Here's how the part is built. I have some questions about the finished solid (model axes, mm). A direction names the side the tool comes from. Give positions to 0.01 mm unless a question says otherwise; leave off trailing zeros. Write each loop counter-clockwise with the first axis right and the second up, starting at its lowest first coordinate (ties: lowest second). Pieces come first, ordered by that corner, then holes. Notation, with made-up numbers: M -39.75,44 L -14.75,44 A9 ccw -14.75,58 Z; hole C -9.75,5.5 d10. An arc over 180 degrees is marked long. Answer as CSV lines item,"result". Start each with the question number.
Q1. Thinking about a two-plate mould opening in Z: for faces 4 (the flat face through (-31, 0, 0)), 5 (the flat face through (-9.891, 12.878, -59.985)), which applies, +Z half, -Z half, draft (parallel to the pull), parting line (faces both ways), or undercut?
Q2. For pin 1 (5 mm diameter, centred on y = 11.5, z = 0, fed in from +X); pin 2 (1 mm diameter, centred on x = -64.5, y = 11, fed in from -Z); pin 3 (10 mm diameter, centred on x = -8, y = 12.5, fed in from +Z), each with a flat end and sliding along its axis, tell me the tip position at first contact or that it passes through.
Q3. Suppose I cut it at A-A (y = 23). Count the separate pieces of the cut face and the enclosed holes in it, then the cut area to 3 significant figures.
Q4. Suppose I cut it at B-B (z = -37.5). Write out the boundary of the cut face in (x, y), then the cut area to 3 significant figures.
Q5. Suppose I cut it at C-C (z = 69.5). Write out the boundary of the cut face in (x, y), then the cut area to 3 significant figures.
Q6. On a 3-axis mill with a long thin cutter (end or side, diameter ignored), from which of +Z, -Z, +X, -X, +Y, -Y can I reach the whole of each face in a straight line? I mean faces 1 (the flat face through (-20, 15, 0)), 2 (the flat face through (-40.752, 12.878, 45.115)), 3 (the cylindrical face through (-5.26, 12.88, -87.24)). Say none if no direction works.
Q7. If I drill on line 1 along X through (y, z) = (14.5, 2); line 2 along X through (y, z) = (3.75, -46.5); line 3 along Z through (x, y) = (-80, 18), over which ranges is the centre line in solid material (lowest first)?
Autodesk Inventor part; units mm, degrees
ref_plane "Work Plane1" through (0, 5, 0) normal (0, 1, 0) x (1, 0, 0)
ref_plane "Work Plane2" through (0, 25.4, 0) normal (0, 1, 0) x (1, 0, 0)
ref_plane "Work Plane3" through (0, 15.4, 0) normal (0, 1, 0) x (1, 0, 0)
sketch "Sketch1" plane through (0, 0, 0) normal (0, 1, 0) x (-1, 0, 0)
  circle A0 centre (0, 0) radius 88.9
  dimension "d0" = 177.8
extrude "Extrusion1" add sketch "Sketch1" along normal blind 25.4
sketch "Sketch2" plane through (0, 25.4, 0) normal (0, 1, 0) x (1, 0, 0)
  circle A0 centre (0, 0) radius 87.4
  line L0 (0, 0) -> (-10.8342, 88.2374)
  circle A1 centre (0, 0) radius 88.9
  line L1 (0, 0) -> (10.8342, 88.2374)
  circle A2 centre (0, 0) radius 34.925
  line L2 (0, 0) -> (0, 88.9)
  point P0 (-4.2563, 34.6647)
  point P1 (4.2563, 34.6647)
  point P2 (10.6514, 86.7485)
  point P3 (-10.6514, 86.7485)
  dimension "d3" = 174.8
  dimension "d4" = 69.85
  dimension "d10" = 14
  dimension "d11" = 7
extrude "Extrusion2" cut sketch "Sketch2" against normal blind 25.4 contours L1 A2 L2 A0 | A0 L2 A2 L0
pattern_circular "Circular Pattern1" count 22 over 360 about axis through (0, 0, 0) along (0, 1, 0) of "Extrusion2"
sketch "Sketch4" plane through (0, 25.4, 0) normal (0, 1, 0) x (1, 0, 0)
  circle A0 centre (0, 0) radius 32.425
  dimension "d16" = 64.85
extrude "Extrusion3" cut sketch "Sketch4" against normal blind 20.4
ref_plane "Work Plane1" through (0, 5, 0) normal (0, 1, 0) x (1, 0, 0)
sketch "Sketch5" plane through (0, 5, 0) normal (0, 1, 0) x (1, 0, 0)
  line L0 (-20, 20) -> (20, 20)
  line L1 (20, 20) -> (20, -20)
  line L2 (20, -20) -> (-20, -20)
  line L3 (-20, -20) -> (-20, 20)
  point P0 (0, 0)
  dimension "d20" = 40
  dimension "d21" = 40
  dimension "d22" = 20
  dimension "d23" = 20
extrude "Extrusion4" add sketch "Sketch5" along normal blind 20.4
ref_plane "Work Plane2" through (0, 25.4, 0) normal (0, 1, 0) x (1, 0, 0)
sketch "Sketch6" plane through (0, 25.4, 0) normal (0, 1, 0) x (1, 0, 0)
  line L0 (-15, 15) -> (15, 15)
  line L1 (15, 15) -> (15, -15)
  line L2 (15, -15) -> (-15, -15)
  line L3 (-15, -15) -> (-15, 15)
  point P0 (0, 0)
  dimension "d26" = 30
  dimension "d27" = 15
  dimension "d28" = 15
  dimension "d29" = 30
extrude "Extrusion5" cut sketch "Sketch6" against normal blind 10
ref_plane "Work Plane3" through (0, 15.4, 0) normal (0, 1, 0) x (1, 0, 0)
sketch "Sketch7" plane through (0, 15.4, 0) normal (0, 1, 0) x (1, 0, 0)
  line L0 (-6, 6) -> (6, 6)
  line L1 (6, 6) -> (6, -6)
  line L2 (6, -6) -> (-6, -6)
  line L3 (-6, -6) -> (-6, 6)
  line L4 (-15, 15) -> (15, 15)
  line L5 (15, 15) -> (15, -15)
  line L6 (-15, -15) -> (-15, 15)
  line L7 (15, -15) -> (-15, -15)
  point P0 (0, 0)
  dimension "d32" = 9
  dimension "d33" = 9
  dimension "d34" = 9
  dimension "d35" = 9
extrude "Extrusion6" cut sketch "Sketch7" against normal blind 10 contours L0 L1 L2 L3
sketch "Sketch16" plane through (0, 0, 0) normal (0, -1, 0) x (1, 0, 0)
  point P0 (0, 0)
ref_plane "Work Plane6" through (0, 25.4, 0) normal (-1, 0, 0) x (0, 0, -1)
sketch "Sketch18" plane through (0, 25.4, 0) normal (-1, 0, 0) x (0, 0, -1)
  line L0 (-99.4236, -8.2024) -> (109.702, -8.2024)
  line L1 (109.702, -8.2024) -> (109.702, 39.2363)
  line L2 (109.702, 39.2363) -> (-99.4236, 39.2363)
  line L3 (-99.4236, 39.2363) -> (-99.4236, -8.2024)
  point P0 (0, 25.4)
extrude "Extrusion7" cut sketch "Sketch18" against normal blind 127
equation "\"d11\" = 0.5 * d10"
equation "\"d21\" = d20"
equation "\"d29\" = d26"
equation "\"d33\" = d32"
equation "\"d34\" = d32"
equation "\"d35\" = d32"
properties part number "Capsule_Design_Final"
Resolved:
1,face 4,"draft"
1,face 5,"undercut"
2,pin 1,"x = -6"
2,pin 2,"z = -61.7"
2,pin 3,"z = 88.85"
3,separate pieces,"2"
3,enclosed holes,"10"
3,area,"2,490 mm^2"
4,outline,"M -80.6,0 L -78.95,0 L -78.95,25.4 L -80.6,25.4 Z; M -61.09,0 L -55.79,0 L -55.79,25.4 L -61.09,25.4 Z; M -33.87,0 L -31.16,0 L -31.16,25.4 L -33.87,25.4 Z; M -18.07,0 L -16.2,0 L -16.2,25.4 L -18.07,25.4 Z; M -6.18,0 L -4.6,0 L -4.6,25.4 L -6.18,25.4 Z"
4,area,"333 mm^2"
5,outline,"M -55.43,0 L -53,0 L -53,25.4 L -55.43,25.4 Z; M -33.49,0 L -30.02,0 L -30.02,25.4 L -33.49,25.4 Z; M -11.46,0 L -8.53,0 L -8.53,25.4 L -11.46,25.4 Z"
5,area,"224 mm^2"
6,face 1,"+Y"
6,face 2,"+Y, -Y"
6,face 3,"+X, +Y, -Y"
7,line 1,"-88.88 to -87.38, -34.87 to -32.36, -20 to -6"
7,line 2,"-75.77 to -69.18, -42 to -38.64, -22.41 to -20.09, -7.67 to -5.71"
7,line 3,"-38.77 to -35.2, -25.29 to -21.71, -1.65 to 1.65, 21.71 to 25.29, 35.2 to 38.77"
